Drawing for the job (mm, zero at the part's lowest x, y, z). Give positions to 0.01 mm unless a question says otherwise; leave off trailing zeros. Order: outer loops, then holes, each group sorted by start corner. A loop starts at its lowest first (then second) coordinate and runs counter-clockwise, first axis right, second up. Notation, with made-up numbers: (41.5, 81.25) -> (56.5, 81.25) arc R10 cw to (56.5, 100.25) -> close; hole circle Ø9 at (-19, 83). An arc over 180 degrees is marked (long way). One line per item, written item: value. Start each with the question number.
(1) Pin check, flat tips, straight feed: pin 1 (8 mm diameter, centred on y = 13, z = 12.5, fed in from +X); pin 2 (12 mm diameter, centred on x = 62.5, y = 55.5, fed in from +Z); pin 3 (4 mm diameter, centred on x = 52.5, z = 22.5, fed in from -Y); pin 4 (5 mm diameter, centred on x = 24, z = 25, fed in from +Y). Stop position of each tip, or through.
(2) Saw through at A-A on z = 6.5. Give the cut face in (x, y).
(3) Probe line 1 (Y direction, x = 43.3, z = 22); line 2 (Y direction, x = 83.3, z = 22.75); line 3 (X direction, y = 46, z = 28.5). List the from-to ranges inside material, lowest first.
(4) Two-plate mould, pull along Y, no slides. Class the marked faces 1 and 2: +Y half, -Y half, draft (parallel to the pull), parting line (faces both ways), or undercut.
(5) Saw through at B-B on y = 33. Give the cut face in (x, z).
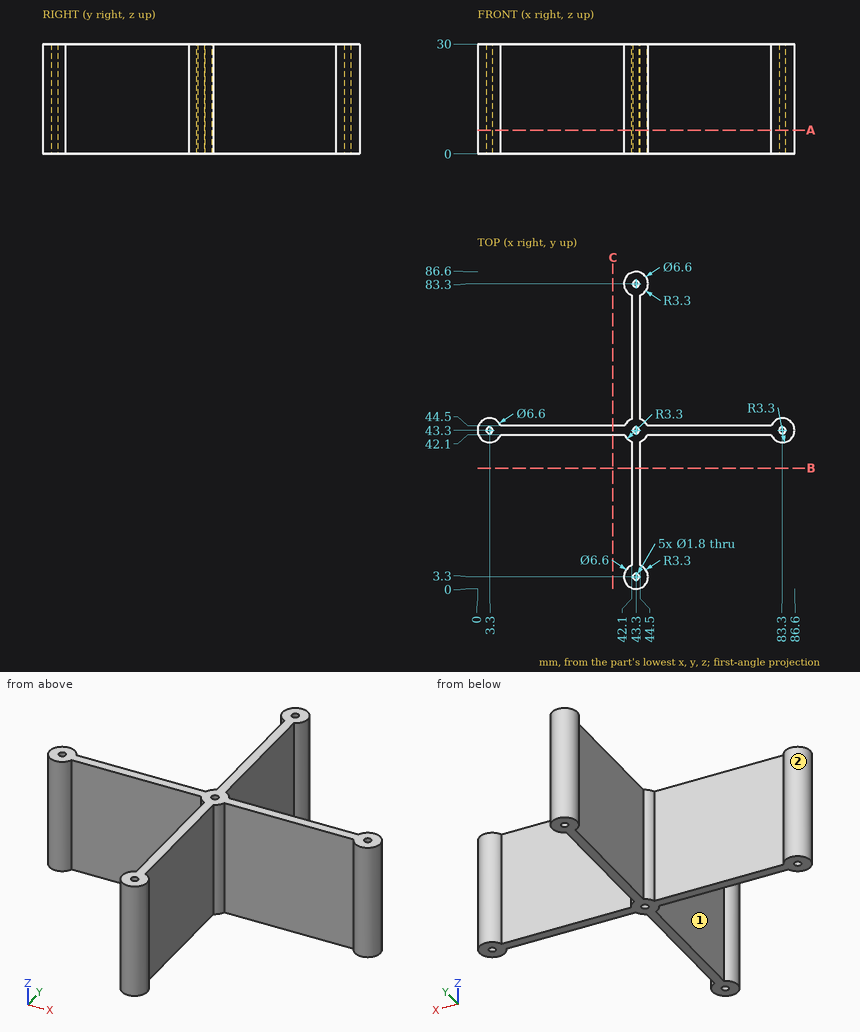
Results below:
1. pin 1: stops at x = 44.5
1. pin 2: passes through
1. pin 3: stops at y = 42.1
1. pin 4: stops at y = 44.5
2. outline: (6.37, 42.1) -> (40.23, 42.1) arc R3.3 ccw to (42.1, 40.23) -> (42.1, 6.37) arc R3.3 ccw (long way) to (44.5, 6.37) -> (44.5, 40.23) arc R3.3 ccw to (46.37, 42.1) -> (80.23, 42.1) arc R3.3 ccw (long way) to (80.23, 44.5) -> (46.37, 44.5) arc R3.3 ccw to (44.5, 46.37) -> (44.5, 80.23) arc R3.3 ccw (long way) to (42.1, 80.23) -> (42.1, 46.37) arc R3.3 ccw to (40.23, 44.5) -> (6.37, 44.5) arc R3.3 ccw (long way) to start; hole circle Ø1.8 at (3.3, 43.3); hole circle Ø1.8 at (43.3, 3.3); hole circle Ø1.8 at (43.3, 43.3); hole circle Ø1.8 at (43.3, 83.3); hole circle Ø1.8 at (83.3, 43.3)
3. line 1: y = 0 to 2.4, 4.2 to 42.4, 44.2 to 82.4, 84.2 to 86.6
3. line 2: y = 40 to 42.4, 44.2 to 46.6
3. line 3: x = 1.4 to 5.2, 41.4 to 45.2, 81.4 to 85.2
4. face 1: undercut
4. face 2: parting line
5. outline: (42.1, 0) -> (44.5, 0) -> (44.5, 30) -> (42.1, 30) -> close
